The model under review builds one solid part; all positions refer to its coordinate system, in mm. A direction names the side the tool comes from. Coordinates: 2 decimals unless noted, no trailing zeros. Answer in a Markdown table with one row per item. Add a question column.
(1) Machinability: for faces 4 (the flat face through (0, 1, 0)), 5 (the flat face through (-2, -20, 1)), which of the approach directions +Z, -Z, +X, -X, +Y, -Y give a long, thin tool a straight path to every point of the face, cutting with its end or side? Answer none if there is none.
(2) For line 1 along X through (y, z) = (-19, 1.5), list the stretches that pass through material, from the lowest coordinate up.
(3) Mouldability with a two-part tool opening along X and no side actions: class faces 1 (the flat face through (-3, -20, 1)), 2 (the flat face through (0, 40, 1)), 3 (the flat face through (27.5, -1, 1)) as +X half, -X half, draft (parallel to the pull), parting line (faces both ways), or undercut.
from build123d import *

# Parameters (mm, degrees)
SKETCH1_W           = 55
SKETCH1_H           = 80
SKETCH1_W_2         = 1
SKETCH1_H_2         = 10
BOSS_EXTRUDE1_DEPTH = 3


with BuildPart() as part:
    # Sketch1 → Boss-Extrude1 (new body)
    with BuildSketch(Plane.XY):
        Rectangle(SKETCH1_W, SKETCH1_H)
        with Locations((2.5, -20)):
            Rectangle(SKETCH1_W_2, SKETCH1_H_2, mode=Mode.SUBTRACT)
        with Locations((-2.5, -20)):
            Rectangle(SKETCH1_W_2, SKETCH1_H_2, mode=Mode.SUBTRACT)
    extrude(amount=BOSS_EXTRUDE1_DEPTH)


solid = part.part
Outcome:
| question | item | result |
|---|---|---|
| 1 | face 4 | -Z, +X, -X, +Y, -Y |
| 1 | face 5 | +Z, -Z |
| 2 | line 1 | -27.5 to -3, -2 to 2, 3 to 27.5 |
| 3 | face 1 | undercut |
| 3 | face 2 | draft |
| 3 | face 3 | +X half |
